Build history of the part. All positions in model axes, mm. Face numbers are marked on the shaded views. A direction names the side the tool comes from. Coordinates: 2 decimals unless noted, no trailing zeros. Order: outer loops, then holes, each group sorted by start corner. A loop starts at its lowest first (then second) coordinate and runs counter-clockwise, first axis right, second up. Notation, with made-up numbers: (-8, 71) - (33, 71) arc R25 ccw to (33, 92) - close; hole circle Ø2 at (15, 45.5). An arc over 180 degrees is marked (long way). Write each question's results on one line, items separated by ' | '.
from build123d import *

# Parameters (mm, degrees)
F0_W     = 431.8
F0_H     = 212.09
F1_DEPTH = 355.6
F2_W     = 414.10742
F2_H     = 338.284008
F3_DEPTH = 205.232
F4_R     = 25.4
F5_DEPTH = 20.066
F6_R     = 12.264205
F7_W     = 42.114318
F7_H     = 11.923939
F8_DEPTH = 76.454


with BuildPart() as f1:
    # F0 (on Front) → F1 (new body)
    with BuildSketch(Plane.XZ):
        Rectangle(F0_W, F0_H)
    extrude(amount=F1_DEPTH)

    # F2 (on face) → F3 (cut)
    with BuildSketch(Plane.XY.offset(106.045)):
        with Locations((-0.196185, -178.056706)):
            Rectangle(F2_W, F2_H)
    extrude(amount=-F3_DEPTH, mode=Mode.SUBTRACT)

    # F4 (on face) → F5 (join)
    with BuildSketch(Plane.XZ.offset(355.6)):
        with Locations((0, 22.440701)):
            Circle(F4_R)
    extrude(amount=F5_DEPTH)

    # F6
    f6_edges = [f1.edges().sort_by_distance(p)[0] for p in [
        (-207.249895, -347.19871, 3.429),
        (-0.196185, -347.19871, -99.187),
        (-207.249895, -178.056706, -99.187),
        (206.857525, -178.056706, -99.187),
        (206.857525, -347.19871, 3.429),
        (-0.196185, -8.914702, -99.187),
        (-207.249895, -8.914702, 3.429),
        (206.857525, -8.914702, 3.429),
    ]]
    fillet(f6_edges, radius=F6_R)

    # F7 (on face) → F8 (cut)
    with BuildSketch(Plane.XY.offset(106.045)):
        with Locations((-0.088485, -366.523399)):
            Rectangle(F7_W, F7_H)
    extrude(amount=-F8_DEPTH, mode=Mode.SUBTRACT)


solid = f1.part
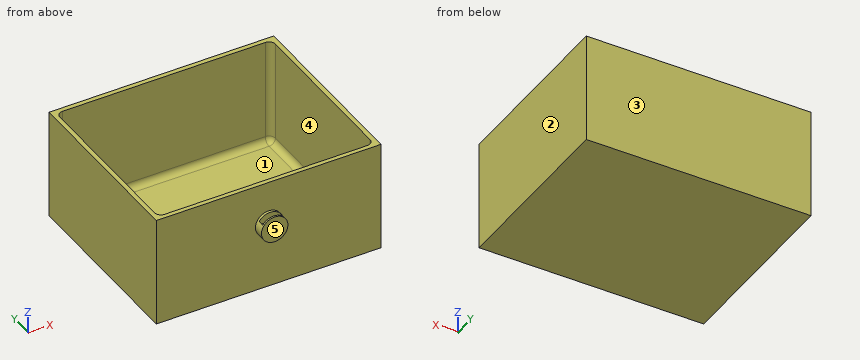
1. Two-plate mould, pull along X, no slides. Class the marked faces 1, 2 and 3: +X half, -X half, draft (parallel to the pull), parting line (faces both ways), or undercut.
Solved:
face 1: undercut | face 2: +X half | face 3: draft
2. Band-saw the part on C-C on y = -274. Give the cut face in (x, z) (3 decimals), then the cut area to 3 significant figures.
Solved:
outline: (-215.9, -106.045) - (215.9, -106.045) - (215.9, 106.045) - (206.858, 106.045) - (206.858, -86.923) arc R12.264 cw to (194.593, -99.187) - (-194.986, -99.187) arc R12.264 cw to (-207.25, -86.923) - (-207.25, 106.045) - (-215.9, 106.045) - close | area: 6,660 mm2
3. Tool access for the marked faces 4 and 5: list every direction of +Z, -Z, +X, -X, +Y, -Y with a clear straight run to the whole face (end or side of a thin tool).
Solved:
face 4: +Z | face 5: +Z, -Z, +X, -X, -Y
4. Probe line 1 (Y direction, x = -50, z = -74); line 2 (X direction, y = -274, z = 60); line 3 (Z direction, x = 173, y = -147) (3 decimals). List the from-to ranges inside material, lowest first.
Solved:
line 1: y = -355.6 to -347.2, -8.91 to 0 | line 2: x = -215.9 to -207.25, 206.86 to 215.9 | line 3: z = -106.045 to -99.187
5. Band-saw the part on B-B on x = 88. Give the cut face in (y, z) (1 decimal), then the cut area to 3 significant figures.
Solved:
outline: (-355.6, -106) - (0, -106) - (0, 106) - (-8.9, 106) - (-8.9, -86.9) arc R12.3 cw to (-21.2, -99.2) - (-334.9, -99.2) arc R12.3 cw to (-347.2, -86.9) - (-347.2, 106) - (-355.6, 106) - close | area: 6,060 mm2
6. Band-saw the part on D-D on x = 0. Give the cut face in (y, z) (1 decimal), then the cut area to 3 significant figures.
Solved:
outline: (-375.7, -3) - (-355.6, -3) - (-355.6, -106) - (0, -106) - (0, 106) - (-8.9, 106) - (-8.9, -86.9) arc R12.3 cw to (-21.2, -99.2) - (-334.9, -99.2) arc R12.3 cw to (-347.2, -86.9) - (-347.2, 106) - (-355.6, 106) - (-355.6, 47.8) - (-360.6, 47.8) - (-360.6, 29.6) - (-372.5, 29.6) - (-372.5, 47.8) - (-375.7, 47.8) - close | area: 6,860 mm2
7. Band-saw the part on A-A on z = -30. Give the cut face in (x, y), then the cut area to 3 significant figures.
Solved:
outline: (-215.9, -355.6) - (215.9, -355.6) - (215.9, 0) - (-215.9, 0) - close; hole (-207.25, -334.93) arc R12.26 ccw to (-194.99, -347.2) - (194.59, -347.2) arc R12.26 ccw to (206.86, -334.93) - (206.86, -21.18) arc R12.26 ccw to (194.59, -8.91) - (-194.99, -8.91) arc R12.26 ccw to (-207.25, -21.18) - close | area: 13,600 mm2
8. Drop flat-ended pins along their axis: pin 1 Ø20 at (x, z) = (-9.5, 39.5) entering from +Y; pin 2 Ø8 at (x, y) = (135, -149) entering from +Z; pin 3 Ø9.5 at (x, y) = (-3.5, -364.5) entering from +Z; pin 4 Ø12 at (x, z) = (-152, 50) entering from -Y. Give the stop position or say it passes through.
Solved:
pin 1: stops at y = 0 | pin 2: stops at z = -99.19 | pin 3: stops at z = 47.83 | pin 4: stops at y = -355.6
